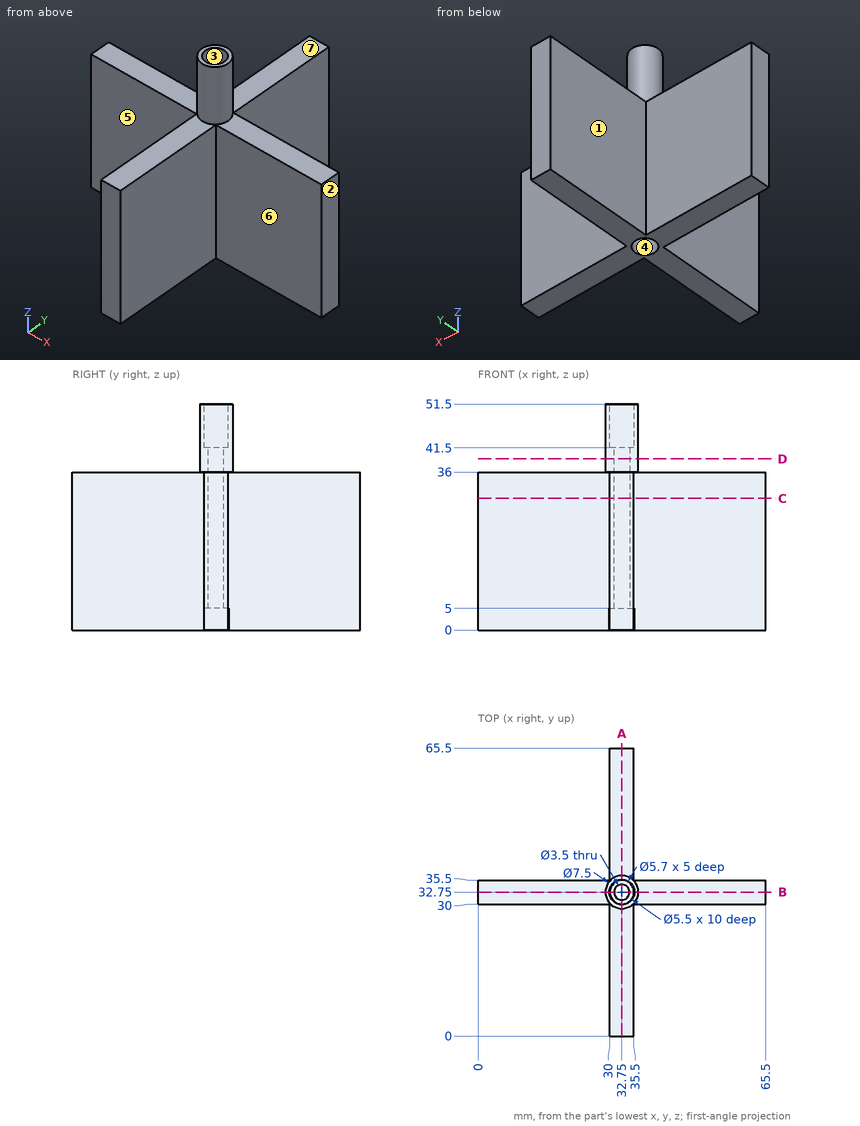
Design review of the part shown in the three views and the two pictorial views. Dimensions are in mm from the part's minimum x, y and z. A direction names the side the tool comes from. Round coordinates to 2 decimals unless told otherwise and drop trailing zeros. Write each loop counter-clockwise with the first axis right and the second up, starting at its lowest first coordinate (ties: lowest second). Pieces come first, ordered by that corner, then holes. Notation, with made-up numbers: (-1.5, 22) -> (30.5, 22) arc R6 ccw to (30.5, 26) -> close; hole circle Ø1 at (68.25, 30.5). An arc over 180 degrees is marked (long way). Use one line per item in the form item = value.
1) Clearance check with flat-ended pins moving along their axes: pin 1 (4.5 mm diameter, centred on x = 33, y = 32.5, fed in from +Z); pin 2 (12 mm diameter, centred on y = 10.5, z = 35, fed in from +X); pin 3 (4 mm diameter, centred on x = 10, z = 29, fed in from -Y); pin 4 (6.5 mm diameter, centred on x = 32.5, y = 33, fed in from -Z). State where each tip first meets the part, or that it passes through.
Found:
pin_1 = 41.5
pin_2 = 35.5
pin_3 = 30
pin_4 = 0
2) Take a section at A-A, the plane x = 32.75. Write out the cut boundary in (y, z).
Found:
outline = (0, 0) -> (29.9, 0) -> (29.9, 5) -> (31, 5) -> (31, 41.5) -> (30, 41.5) -> (30, 51.5) -> (29, 51.5) -> (29, 36) -> (0, 36) -> close; (34.5, 5) -> (35.6, 5) -> (35.6, 0) -> (65.5, 0) -> (65.5, 36) -> (36.5, 36) -> (36.5, 51.5) -> (35.5, 51.5) -> (35.5, 41.5) -> (34.5, 41.5) -> close
3) Take a section at C-C, the plane z = 30. Write out the cut boundary in (x, y), and give its area (3 significant figures).
Found:
outline = (0, 30) -> (30, 30) -> (30, 0) -> (35.5, 0) -> (35.5, 30) -> (65.5, 30) -> (65.5, 35.5) -> (35.5, 35.5) -> (35.5, 65.5) -> (30, 65.5) -> (30, 35.5) -> (0, 35.5) -> close; hole circle Ø3.5 at (32.75, 32.75)
area = 681 mm2
4) Tool access review of the marked faces 5, 6 and 7: name each direction out of +Z, -Z, +X, -X, +Y, -Y from which nothing blocks a thin tool from reaching the whole face with its end or side.
Found:
face_5 = +Z, -Z, -X, -Y
face_6 = +Z, -Z, +X, -Y
face_7 = +Z
5) Take a section at D-D, the plane z = 39. Write out the cut boundary in (x, y).
Found:
outline = circle Ø7.5 at (32.75, 32.75); hole circle Ø3.5 at (32.75, 32.75)
6) Mouldability with a two-part tool opening along X and no side actions: class the marked faces 1, 2, 3 and 4 as +X half, -X half, draft (parallel to the pull), parting line (faces both ways), or undercut.
Found:
face_1 = -X half
face_2 = +X half
face_3 = undercut
face_4 = undercut
7) To check wall thickness, follow L1, parallel to Y at x = 32, z = 2; L2, parallel to X at y = 32.5, z = 37. State the ranges of each line that lie inside material, in increasing order. Write a range as from..to.
Found:
L1 = 0..30, 35.5..65.5
L2 = 29.01..31.02, 34.48..36.49
